Build history of the part. All positions in model axes, mm. Give positions to 0.01 mm unless a question says otherwise; leave off trailing zeros. Loops run counter-clockwise (first coordinate to the right, second up) from the corner with the lowest first, then second, coordinate; pieces in that order, holes last. Notation, with made-up numbers: (-5.75, -9) -> (30.25, -9) arc R11 cw to (30.25, 4) -> close; hole circle Ø10 at (-7.5, -12). An arc over 180 degrees is marked (long way). Answer as a JSON object with one key per item and string values. Group by question number.
Q1. Wall check: probe 1 along X at (y, z) = (0.05, 0.9); probe 2 along X at (y, z) = (0.65, 0.65); probe 3 along Y at (x, z) = (0, 1.45). Give the ranges that are in metal, low to high. Write a range as from..to.
Q2. Two-plate mould, pull along Y, no slides. Class faces 1 (the cylindrical face through (16, 0, 1)), 2 (the flat face through (7, -2.5, 1)), 3 (the flat face through (7, 0, 0)): pulls with the +Y half, pulls with the -Y half, needs draft (parallel to the pull), parting line crosses it, or undercut.
Q3. Band-saw the part on A-A, the plane y = 0. Write the cut outline in (x, z).
Q4. Band-saw the part on B-B, the plane z = 0.75. Write the cut outline in (x, y).
Autodesk Inventor part; units mm, degrees
ref_plane "YZ Plane" through (0, 0, 0) normal (1, 0, 0) x (0, 1, 0)
ref_plane "XZ Plane" through (0, 0, 0) normal (0, 1, 0) x (-1, 0, 0)
ref_plane "XY Plane" through (0, 0, 0) normal (0, 0, 1) x (1, 0, 0)
sketch "Sketch1" plane through (0, 0, 0) normal (0, 0, 1) x (1, 0, 0)
  line L0 (0, 0) -> (15, 0) construction
  line L1 (0, -2.5) -> (15, -2.5)
  line L2 (15, 2.5) -> (0, 2.5)
  arc A0 (0, 2.5) -> (0, -2.5) centre (0, 0) ccw
  arc A1 (15, -2.5) -> (15, 2.5) centre (15, 0) ccw
  circle A2 centre (15, 0) radius 1
  circle A3 centre (0, 0) radius 1
  point P0 (7.5, 0)
  dimension "d0" = 15
  dimension "d1" = 5
  dimension "d2" = 2
  dimension "d3" = 2
extrude "Extrusion1" add sketch "Sketch1" along normal blind 2
sketch "Sketch2" plane through (0, 0, 2) normal (0, 0, 1) x (1, 0, 0)
  circle A0 centre (0, 0) radius 0.75
  circle A1 centre (0, 0) radius 1
  dimension "d6" = 1.5
extrude "Extrusion2" add sketch "Sketch2" against normal blind 2
properties part number "horn slider pen"
Worked answers:
{
 "1": {"probe 1": "-2.5..-0.75, 0.75..14, 16..17.5", "probe 2": "-2.41..-0.37, 0.37..14.24, 15.76..17.41", "probe 3": "-2.5..-0.75, 0.75..2.5"},
 "2": {"face 1": "undercut", "face 2": "pulls with the -Y half", "face 3": "needs draft"},
 "3": {"outline": "(-2.5, 0) -> (-0.75, 0) -> (-0.75, 2) -> (-2.5, 2) -> close; (0.75, 0) -> (14, 0) -> (14, 2) -> (0.75, 2) -> close; (16, 0) -> (17.5, 0) -> (17.5, 2) -> (16, 2) -> close"},
 "4": {"outline": "(0, -2.5) -> (15, -2.5) arc R2.5 ccw to (15, 2.5) -> (0, 2.5) arc R2.5 ccw to start; hole circle Ø1.5 at (0, 0); hole circle Ø2 at (15, 0)"}
}
